CAD build for the part. Positions are in the model's coordinates, mm. Face numbers are marked on the shaded views. Give positions to 0.01 mm unless a question says otherwise; leave off trailing zeros. Order: outer loops, then holes, each group sorted by start corner. A loop starts at its lowest first (then second) coordinate and runs counter-clockwise, first axis right, second up. Notation, with made-up numbers: (44, 60.25) -> (61, 60.25) arc R14 cw to (61, 84.25) -> close; hole circle Ø11 at (-34.5, 2.5). An arc over 180 degrees is marked (long way). Answer as CSV lines item,"result".
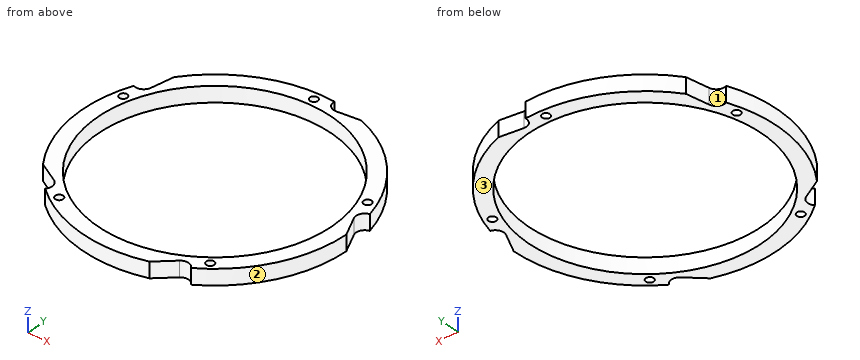
Autodesk Inventor part; units mm, degrees
ref_plane "YZ Plane" through (0, 0, 0) normal (1, 0, 0) x (0, 1, 0)
ref_plane "XZ Plane" through (0, 0, 0) normal (0, 1, 0) x (-1, 0, 0)
ref_plane "XY Plane" through (0, 0, 0) normal (0, 0, 1) x (1, 0, 0)
sketch "Sketch1" plane through (0, 0, 0) normal (0, 0, 1) x (1, 0, 0)
  circle A0 centre (77.3169, -37.9173) radius 75
  circle A1 centre (77.3169, -37.9173) radius 85
  circle A2 centre (77.3169, -37.9173) radius 75
  point P0 (0, 0)
  dimension "d0" = 150
  dimension "d1" = 170
extrude "Extrusion1" add sketch "Sketch1" along normal blind 10
sketch "Sketch3" plane through (77.3169, -37.9173, 10) normal (0, 0, 1) x (1, 0, 0)
  circle A0 centre (-76.5194, 37.0443) radius 2.5 construction
  circle A1 centre (-58.877, -61.3269) radius 2.5 construction
  circle A2 centre (40.1314, -74.9464) radius 2.5 construction
  circle A3 centre (83.6796, 15.0075) radius 2.5 construction
  circle A4 centre (11.5854, 84.2216) radius 2.5 construction
  line L0 (40.1314, -74.9464) -> (25.5443, -88.6291) construction
  line L1 (36.3686, -70.935) -> (21.7815, -84.6177)
  line L2 (29.307, -92.6406) -> (43.8941, -78.9579)
  arc A5 (43.8941, -78.9579) -> (36.3686, -70.935) centre (40.1314, -74.9464) ccw
  arc A6 (21.7815, -84.6177) -> (29.307, -92.6406) centre (25.5443, -88.6291) ccw
  line L3 (40.1314, -74.9464) -> (48.951, -91.4173) construction
  circle A7 centre (0, 0) radius 85 construction
  line L4 (78.7017, 12.6685) -> (87.207, -5.4328)
  line L5 (97.1628, -0.7549) -> (88.6574, 17.3465)
  arc A8 (88.6574, 17.3465) -> (78.7017, 12.6685) centre (83.6796, 15.0075) ccw
  arc A9 (87.207, -5.4328) -> (97.1628, -0.7549) centre (92.1849, -3.0939) ccw
  line L6 (12.2717, 78.7645) -> (32.1154, 81.26)
  line L7 (30.7429, 92.174) -> (10.8992, 89.6786)
  arc A10 (10.8992, 89.6786) -> (12.2717, 78.7645) centre (11.5854, 84.2216) ccw
  arc A11 (32.1154, 81.26) -> (30.7429, 92.174) centre (31.4292, 86.717) ccw
  line L8 (-71.1174, 36.0107) -> (-67.3586, 55.6543)
  line L9 (-78.1626, 57.7216) -> (-81.9214, 38.078)
  arc A12 (-81.9214, 38.078) -> (-71.1174, 36.0107) centre (-76.5194, 37.0443) ccw
  arc A13 (-67.3586, 55.6543) -> (-78.1626, 57.7216) centre (-72.7606, 56.6879) ccw
  line L10 (-56.2246, -56.5087) -> (-73.7453, -46.8638)
  line L11 (-79.0501, -56.5001) -> (-61.5294, -66.1451)
  arc A14 (-61.5294, -66.1451) -> (-56.2246, -56.5087) centre (-58.877, -61.3269) ccw
  arc A15 (-73.7453, -46.8638) -> (-79.0501, -56.5001) centre (-76.3977, -51.6819) ccw
  point P0 (-77.3169, 37.9173)
  point P1 (32.8378, -81.7878)
  dimension "d22" = 11
  dimension "d23" = 75
  dimension "d24" = 20
  dimension "d27" = 360
extrude "Extrusion5" cut sketch "Sketch3" against normal blind 10
sketch "Sketch4" plane through (0, 0, 10) normal (0, 0, 1) x (1, 0, 0)
  circle A0 centre (0.3478, -16.1054) radius 2.5
  circle A1 centre (32.7878, -104.379) radius 2.5
  circle A2 centre (126.7655, -100.8047) radius 2.5
  circle A3 centre (152.4069, -10.3221) radius 2.5
  circle A4 centre (74.2765, 42.0249) radius 2.5
  point P0 (0, 0)
hole "Hole1" at (32.7878, -104.379, 10) at (126.7655, -100.8047, 10) at (152.4069, -10.3221, 10) at (74.2765, 42.0249, 10) at (0.3478, -16.1054, 10) direction (0, 0, -1) diameter 5 end through all
properties part number "innerring"
1) Wall check: line 1 along X through (y, z) = (-16.5, 2.75); line 2 along Y through (x, z) = (35, 5); line 3 along X through (y, z) = (-106.5, 2.75). Give the ranges that are in metal, low to high. Write a range as [from, to].
Data:
line 1,"x = [-4.94, -2.12], [2.82, 5.44], [149.19, 159.57]"
line 2,"y = [-111.63, -105.54], [-103.21, -99.84], [24, 35.8]"
line 3,"x = [27.1, 31.46], [34.11, 46.96], [107.67, 127.53]"
2) Pull direction X, two halves, no side cores. Call the marked faces 1, 2 and 3: pulls with the +X half, pulls with the -X half, needs draft (parallel to the pull), parting line crosses it, or undercut.
Data:
face 1,"undercut"
face 2,"pulls with the +X half"
face 3,"needs draft"
3) Band-saw the part on C-C, the plane z = 8.25. Write the cut outline in (x, y), then the cut area to 3 significant figures.
Data:
outline,"(-1.42, -5.9) arc R85 ccw to (8.12, -87.29) -> (21.09, -94.43) arc R5.5 cw to (22.54, -102.91) arc R85 ccw to (102.89, -118.98) -> (113.69, -108.85) arc R5.5 cw to (122.2, -110.1) arc R85 ccw to (162.31, -38.65) -> (156.02, -25.25) arc R5.5 cw to (159.84, -17.53) arc R85 ccw to (104.28, 42.69) -> (89.59, 40.85) arc R5.5 cw to (83.43, 46.86) arc R85 ccw to (8.98, 12.63) -> (6.2, -1.91) arc R5.5 cw to start; hole circle Ø5 at (0.35, -16.11); hole circle Ø150 at (77.32, -37.92); hole circle Ø5 at (32.79, -104.38); hole circle Ø5 at (74.28, 42.02); hole circle Ø5 at (126.77, -100.8); hole circle Ø5 at (152.41, -10.32)"
area,"4,570 mm2"
4) Band-saw the part on B-B, the plane y = -91.5. Write the cut outline in (x, z).
Data:
outline,"(15.78, 0) -> (24.84, 0) -> (24.84, 10) -> (15.78, 10) -> close; (129.79, 0) -> (143.3, 0) -> (143.3, 10) -> (129.79, 10) -> close"
5) Band-saw the part on A-A, the plane x = 100. Write the cut outline in (y, z), then the cut area to 3 significant figures.
Data:
outline,"(-119.83, 0) -> (-109.4, 0) -> (-109.4, 10) -> (-119.83, 10) -> close; (33.57, 0) -> (42.16, 0) -> (42.16, 10) -> (33.57, 10) -> close"
area,"190 mm2"
6) Pin check, flat tips, straight feed: P1, Ø10, axis at x = 57.5, y = -100, coming from the -Z side; P2, Ø6, axis at y = -104.5, z = 7.5, coming from the -X side; P3, Ø2, axis at y = -1, z = 5.5, coming from the -X side. Stop position of each tip, or through.
Data:
P1,"passes through"
P2,"stops at x = 22.54"
P3,"stops at x = 6.18"
